from build123d import *

# Parameters (mm, degrees)
SKETCH1_R           = 26.590625
BOSS_EXTRUDE1_DEPTH = 1.5875
SKETCH2_R           = 25.5984375
BOSS_EXTRUDE2_DEPTH = 2.38125
SKETCH3_R           = 26.590625
BOSS_EXTRUDE3_DEPTH = 1.5875
SKETCH5_R           = 14.2875
BOSS_EXTRUDE4_DEPTH = 0.79375
SKETCH6_R           = 11.1125
CUT_EXTRUDE1_DEPTH  = 39.137188881
FILLET1_R           = 1
FILLET2_R           = 1


with BuildPart() as part:
    # Sketch1 → Boss-Extrude1 (new body)
    with BuildSketch(Plane(origin=(0, 0, 0), x_dir=(1, 0, 0), z_dir=(0, 1, 0))):
        with Locations(Location((0, 0, 0), (0, 0, 270))):
            Circle(SKETCH1_R)
    extrude(amount=BOSS_EXTRUDE1_DEPTH)

    # Sketch2 → Boss-Extrude2 (add)
    with BuildSketch(Plane(origin=(0, 1.5875, 0), x_dir=(1, 0, 0), z_dir=(0, 1, 0))):
        with Locations(Location((0, 0, 0), (0, 0, 90))):
            Circle(SKETCH2_R)
    extrude(amount=BOSS_EXTRUDE2_DEPTH)

    # Sketch3 → Boss-Extrude3 (add)
    with BuildSketch(Plane(origin=(0, 3.96875, 0), x_dir=(1, 0, 0), z_dir=(0, 1, 0))):
        with Locations(Location((0, 0, 0), (0, 0, 270))):
            Circle(SKETCH3_R)
    extrude(amount=BOSS_EXTRUDE3_DEPTH)

    # Sketch5 → Boss-Extrude4 (add)
    with BuildSketch(Plane(origin=(0, 5.55625, 0), x_dir=(1, 0, 0), z_dir=(0, 1, 0))):
        with Locations(Location((0, 0, 0), (0, 0, 270))):
            Circle(SKETCH5_R)
    extrude(amount=BOSS_EXTRUDE4_DEPTH)

    # Sketch6 → Cut-Extrude1 (cut, through all)
    with BuildSketch(Plane(origin=(0, 6.35, 0), x_dir=(1, 0, 0), z_dir=(0, 1, 0))):
        with Locations(Location((0, 0, 0), (0, 0, 270))):
            Circle(SKETCH6_R)
    extrude(amount=-CUT_EXTRUDE1_DEPTH, mode=Mode.SUBTRACT)

    # Fillet1
    # the kernel refuses this fillet: 1 mm, written as the material it adds along each edge
    with BuildSketch(Plane(origin=(0, 1.5875, 0), x_dir=(0, 0, -1), z_dir=(1, 0, 0))) as fillet1_piece_1_section:
        with BuildLine():
            CenterArc((25.5984375 + FILLET1_R, FILLET1_R), FILLET1_R, 180, 90)
            Line((25.5984375 + FILLET1_R, 0), (25.5984375, 0))
            Line((25.5984375, 0), (25.5984375, FILLET1_R))
        make_face()
    fillet1_piece_1 = revolve(axis=Axis((0, 1.5875, 0), (0, 1, 0)), mode=Mode.PRIVATE)
    fillet1_piece_1 = fillet1_piece_1 & Plane(origin=(0, 1.858804506, 0), x_dir=(0, 0, 1), z_dir=(0, -1, 0)) * Cylinder(26.590625, 107, mode=Mode.PRIVATE)
    add(fillet1_piece_1)

    # Fillet2
    # the kernel refuses this fillet: 1 mm, written as the material it adds along each edge
    with BuildSketch(Plane(origin=(0, 3.96875, 0), x_dir=(0, 0, -1), z_dir=(1, 0, 0))) as fillet2_piece_1_section:
        with BuildLine():
            CenterArc((25.5984375 + FILLET2_R, -FILLET2_R), FILLET2_R, 90, 90)
            Line((25.5984375 + FILLET2_R, 0), (25.5984375, 0))
            Line((25.5984375, 0), (25.5984375, -FILLET2_R))
        make_face()
    fillet2_piece_1 = revolve(axis=Axis((0, 3.96875, 0), (0, 1, 0)), mode=Mode.PRIVATE)
    fillet2_piece_1 = fillet2_piece_1 & Plane(origin=(0, 3.697445494, 0), x_dir=(0, 0, 1), z_dir=(0, -1, 0)) * Cylinder(26.590625, 107, mode=Mode.PRIVATE)
    add(fillet2_piece_1)


solid = part.part
The listing builds one solid part. Answer for the finished solid, in the listing's coordinates (mm). Give positions to 0.01 mm unless a question says otherwise; leave off trailing zeros. Loops run counter-clockwise (first coordinate to the right, second up) from the corner with the lowest first, then second, coordinate; pieces in that order, holes last. Notation, with made-up numbers: (55.25, 65) - (110.25, 65) arc R15 ccw to (110.25, 88) - close; hole circle Ø7 at (-23.75, -37.75). An arc over 180 degrees is marked (long way). Write each question's results on one line, items separated by ' | '.
1. For a pull along Y with two mould halves and no side action, classify faces 1 (the face through (-11.4, 0, -0.4)), 2 (the face through (22.71, 2.78, -11.81)), 3 (the face through (0.628, 5.948, -14.274)), 4 (the face through (-11, 5.556, 11)) as +Y half, -Y half, draft (parallel to the pull), parting line (faces both ways), or undercut.
Resolved:
face 1: -Y half | face 2: undercut | face 3: draft | face 4: +Y half
2. Find section B-B, the plane z = 0. Write down the section's boundary in (x, y), then the cut area to 3 significant figures.
Resolved:
outline: (-26.59, 0) - (-11.11, 0) - (-11.11, 6.35) - (-14.29, 6.35) - (-14.29, 5.56) - (-26.59, 5.56) - (-26.59, 3.97) arc R1 cw to (-25.6, 2.97) - (-25.6, 2.59) arc R1 cw to (-26.59, 1.59) - close; (11.11, 0) - (26.59, 0) - (26.59, 1.59) arc R1 cw to (25.6, 2.59) - (25.6, 2.97) arc R1 cw to (26.59, 3.97) - (26.59, 5.56) - (14.29, 5.56) - (14.29, 6.35) - (11.11, 6.35) - close | area: 173 mm^2
3. Find section A-A, the plane x = 0. Write down the section's boundary in (y, z).
Resolved:
outline: (0, -26.59) - (1.59, -26.59) arc R1 cw to (2.59, -25.6) - (2.97, -25.6) arc R1 cw to (3.97, -26.59) - (5.56, -26.59) - (5.56, -14.29) - (6.35, -14.29) - (6.35, -11.11) - (0, -11.11) - close; (0, 11.11) - (6.35, 11.11) - (6.35, 14.29) - (5.56, 14.29) - (5.56, 26.59) - (3.97, 26.59) arc R1 cw to (2.97, 25.6) - (2.59, 25.6) arc R1 cw to (1.59, 26.59) - (0, 26.59) - close
4. Flat-ended cylindrical pins translate along their axes: P1, Ø1.5, axis at y = 3, z = -15, coming from the -X side; P2, Ø3, axis at x = -20.5, y = 4.5, coming from the +Z side; P3, Ø1.5, axis at x = 3.5, y = 4.5, coming from the -Z side. Find the tip coordinate at first contact, or state that the pin passes through.
Resolved:
P1: stops at x = -21.33 | P2: stops at z = 18.6 | P3: stops at z = -26.45
5. Consider probe 1 along X at (y, z) = (4.75, 0); probe 2 along X at (y, z) = (2.75, 0); probe 3 along Y at (x, z) = (16, -10). Determine where each line is inside the solid, lowest interval first. Write a range as from..to.
Resolved:
probe 1: x = -26.59..-11.11, 11.11..26.59 | probe 2: x = -25.6..-11.11, 11.11..25.6 | probe 3: y = 0..5.56
